from build123d import *

# Parameters (mm, degrees)
SKETCH1_R                = 30
SKETCH1_R_2              = 2
BOSS_EXTRUDE1_DEPTH      = 2
SKETCH3_R                = 1
CUT_EXTRUDE1_DEPTH       = 3
SKETCH4_R                = 2
CUT_EXTRUDE2_DEPTH       = 10
FILLET1_R                = 2
CIRPATTERN1_COUNT        = 3
FILLET1_OF_CIRPATTERN1_R = 2


with BuildPart() as part:
    # Sketch1 → Boss-Extrude1 (new body)
    with BuildSketch(Plane(origin=(0, 0, 0), x_dir=(1, 0, 0), z_dir=(0, 1, 0))):
        with Locations(Location((0, 0, 0), (0, 0, 270))):
            Circle(SKETCH1_R)
        with Locations(Location((0, 27, 0), (0, 0, 270))):
            Circle(SKETCH1_R_2, mode=Mode.SUBTRACT)
        with Locations(Location((23.382685902, 13.5, 0), (0, 0, 270))):
            Circle(SKETCH1_R_2, mode=Mode.SUBTRACT)
        with Locations(Location((23.382685902, -13.5, 0), (0, 0, 270))):
            Circle(SKETCH1_R_2, mode=Mode.SUBTRACT)
        with Locations(Location((0, -27, 0), (0, 0, 270))):
            Circle(SKETCH1_R_2, mode=Mode.SUBTRACT)
        with Locations(Location((-23.382685902, -13.5, 0), (0, 0, 270))):
            Circle(SKETCH1_R_2, mode=Mode.SUBTRACT)
        with Locations(Location((-23.382685902, 13.5, 0), (0, 0, 270))):
            Circle(SKETCH1_R_2, mode=Mode.SUBTRACT)
    extrude(amount=BOSS_EXTRUDE1_DEPTH)

    # Sketch3 → Cut-Extrude1 (cut)
    with BuildSketch(Plane(origin=(0, 2, 0), x_dir=(1, 0, 0), z_dir=(0, 1, 0))):
        with Locations(Location((-13.5, 23.382685902, 0), (0, 0, 270))):
            Circle(SKETCH3_R)
        with Locations(Location((13.5, 23.382685902, 0), (0, 0, 270))):
            Circle(SKETCH3_R)
        with Locations(Location((27, 0, 0), (0, 0, 270))):
            Circle(SKETCH3_R)
        with Locations(Location((13.5, -23.382685902, 0), (0, 0, 270))):
            Circle(SKETCH3_R)
        with Locations(Location((-13.5, -23.382685902, 0), (0, 0, 270))):
            Circle(SKETCH3_R)
        with Locations(Location((-27, 0, 0), (0, 0, 270))):
            Circle(SKETCH3_R)
    extrude(amount=-CUT_EXTRUDE1_DEPTH, mode=Mode.SUBTRACT)

    # Sketch4 → Cut-Extrude2 (cut)
    with BuildSketch(Plane(origin=(0, 2, 0), x_dir=(1, 0, 0), z_dir=(0, 1, 0))):
        with Locations(Location((0, 0, 0), (0, 0, 270))):
            Circle(SKETCH4_R)
        with BuildLine():
            Line((-1.09088921, 3.848371179), (-14.680142304, 17.051200014))
            ThreePointArc((-14.680142304, 17.051200014), (5.509393992, 21.815053927), (21.015954319, 8.036147338))
            Line((21.015954319, 8.036147338), (2.787342599, 2.868923358))
            ThreePointArc((2.787342599, 2.868923358), (0.979447821, 3.878231809), (-1.09088921, 3.848371179))
        make_face()
    cut_extrude2 = extrude(amount=-CUT_EXTRUDE2_DEPTH, mode=Mode.SUBTRACT)

    # Fillet1
    fillet1_edges = [part.edges().sort_by_distance(p)[0] for p in [
        (2.787342599, 1, -2.868923358),
        (-1.09088921, 1, -3.848371179),
        (-14.680142304, 1, -17.051200014),
        (21.015954319, 1, -8.036147338),
    ]]
    fillet(fillet1_edges, radius=FILLET1_R)

    # CirPattern1: Cut-Extrude2 ×3 about axis
    cirpattern1_axis = Axis((0, 0, 0), (0, 1, 0))
    for i in range(1, CIRPATTERN1_COUNT):
        add(cut_extrude2.rotate(cirpattern1_axis, i * 360 / CIRPATTERN1_COUNT), mode=Mode.SUBTRACT)

    # Fillet1 of CirPattern1
    fillet1_of_cirpattern1_edges = [part.edges().sort_by_distance(p)[0] for p in [
        (-3.878231809, 1, -0.979447821),
        (-2.787342599, 1, 2.868923358),
        (-7.426701225, 1, 21.238976174),
        (-17.467484903, 1, -14.182276656),
        (1.09088921, 1, 3.848371179),
        (3.878231809, 1, 0.979447821),
        (22.10684353, 1, -4.187776159),
        (-3.548469416, 1, 22.218423995),
    ]]
    fillet(fillet1_of_cirpattern1_edges, radius=FILLET1_OF_CIRPATTERN1_R)


solid = part.part
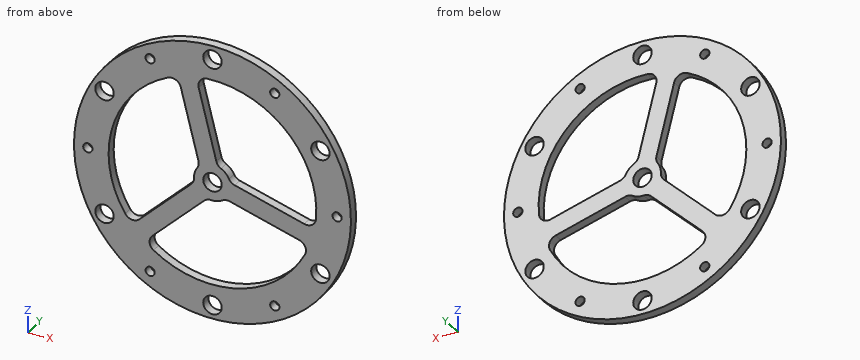
Design review of the part built by this model. Coordinates are the model's own, in mm. Coordinates: 2 decimals unless noted, no trailing zeros. Loops run counter-clockwise (first coordinate to the right, second up) from the corner with the lowest first, then second, coordinate; pieces in that order, holes last.
Item 1: Add section B-B (x = -27). Write out the cut boundary in (y, z).
Completed:
outline: (0, -13.08) - (2, -13.08) - (2, -1) - (0, -1) - close; (0, 1) - (2, 1) - (2, 13.08) - (0, 13.08) - close
Item 2: Add section A-A (z = 17.5). Write out the cut boundary in (x, y).
Completed:
outline: (-24.37, 0) - (-14.14, 0) - (-14.14, 2) - (-24.37, 2) - close; (-6.48, 0) - (-2.36, 0) - (-2.36, 2) - (-6.48, 2) - close; (14.14, 0) - (24.37, 0) - (24.37, 2) - (14.14, 2) - close
Item 3: Add section D-D (z = -27). Write out the cut boundary in (x, y).
Completed:
outline: (-13.08, 0) - (-2, 0) - (-2, 2) - (-13.08, 2) - close; (2, 0) - (13.08, 0) - (13.08, 2) - (2, 2) - close
Item 4: Add section C-C (x = 6). Write out the cut boundary in (y, z).
Completed:
outline: (0, -29.39) - (2, -29.39) - (2, -21.69) - (0, -21.69) - close; (0, -3.78) - (2, -3.78) - (2, 0.38) - (0, 0.38) - close; (0, 21.69) - (2, 21.69) - (2, 29.39) - (0, 29.39) - close
Item 5: Wall thickness on L1, parallel to Z at x = 4, y = 0.35; L2, parallel to Z at x = 3, y = 0.7; L3, parallel to X at y = 1.95, z = 10: over which ranges is each line inside the solid? List them lowest first.
Completed:
L1: z = -29.73 to -22.14, -3.21 to 1.19, 22.14 to 29.73
L2: z = -29.85 to -22.3, -3.08 to 2.65, 22.3 to 29.85
L3: x = -28.28 to -20.16, -4.59 to -0.46, 20.16 to 28.28
